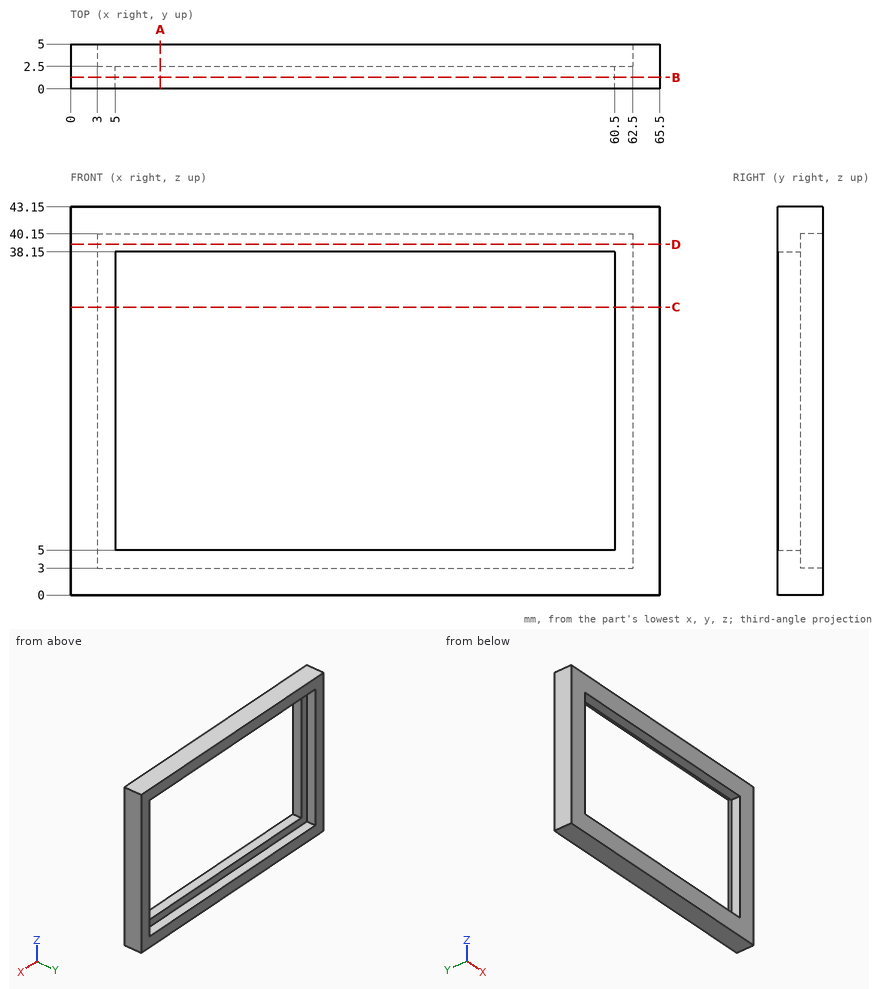
Print and shaded views of the part. All mm, measured from the part's lowest x, y and z. Coordinates: 2 decimals unless noted, no trailing zeros. Order: outer loops, then holes, each group sorted by start corner. A loop starts at its lowest first (then second) coordinate and runs counter-clockwise, first axis right, second up.
(1) Pin check, flat tips, straight feed: pin 1 Ø8 at (x, z) = (7.5, 8) entering from +Y; pin 2 Ø0.8 at (y, z) = (1, 28.5) entering from -X. Stop position of each tip, or through.
Check sheet entries:
pin 1: stops at y = 2.5
pin 2: stops at x = 0
(2) Probe L1, parallel to X at y = 1.7, z = 12.5; L2, parallel to Z at x = 59, y = 2.55; L3, parallel to Z at x = 25, y = 1.1. List the from-to ranges inside material, lowest first.
Check sheet entries:
L1: x = 0 to 5, 60.5 to 65.5
L2: z = 0 to 3, 40.15 to 43.15
L3: z = 0 to 5, 38.15 to 43.15
(3) Slice it at C-C, the plane z = 32. Write the cut outline in (x, y), and give its area (3 significant figures).
Check sheet entries:
outline: (0, 0) - (5, 0) - (5, 2.5) - (3, 2.5) - (3, 5) - (0, 5) - close; (60.5, 0) - (65.5, 0) - (65.5, 5) - (62.5, 5) - (62.5, 2.5) - (60.5, 2.5) - close
area: 40.0 mm2
(4) Slice it at D-D, the plane z = 39. Write the cut outline in (x, y).
Check sheet entries:
outline: (0, 0) - (65.5, 0) - (65.5, 5) - (62.5, 5) - (62.5, 2.5) - (3, 2.5) - (3, 5) - (0, 5) - close
(5) Slice it at A-A, the plane x = 10. Write the cut outline in (y, z), and give its area (3 significant figures).
Check sheet entries:
outline: (0, 0) - (5, 0) - (5, 3) - (2.5, 3) - (2.5, 5) - (0, 5) - close; (0, 38.15) - (2.5, 38.15) - (2.5, 40.15) - (5, 40.15) - (5, 43.15) - (0, 43.15) - close
area: 40.0 mm2
(6) Slice it at B-B, the plane y = 1.3. Write the cut outline in (x, z), and give its area (4 significant figures).
Check sheet entries:
outline: (0, 0) - (65.5, 0) - (65.5, 43.15) - (0, 43.15) - close; hole (5, 5) - (60.5, 5) - (60.5, 38.15) - (5, 38.15) - close
area: 986.5 mm2
